Can you work these out from the model? Positions are in its coordinate system, mm. A direction names the side the tool comes from. Give positions to 0.01 mm unless a question says otherwise; leave off trailing zeros. Loops run counter-clockwise (first coordinate to the right, second up) from the corner with the lowest first, then second, coordinate; pieces in that order, holes last. Notation, with made-up numbers: M 17.25,-22 L 43.25,-22 A29 cw 43.25,-1 Z; hole C 48,69 d11. An arc over 180 degrees is marked long. One line per item, written item: value. Start each with the question number.
from build123d import *

# Parameters (mm, degrees)
F1_DEPTH    = 40.894
F2_R        = 5.08
F3_T1_DEPTH = 52.2452971888
F3_S5_W     = 5.08
F3_S5_H     = 5.08
F3_T6_DEPTH = 5.08
F4_W        = 7.728997618
F4_H        = 30.734
F4_W_2      = 7.9892426729
F5_DEPTH    = 5.08
F6_W        = 4.2550079525
F6_H        = 3.1596273184
F6_W_2      = 3.8497596979
F6_H_2      = 2.54
F7_DEPTH    = 39.37


# Not quite as in the source:
# - a fillet or chamfer that OpenCascade refuses, or shapes differently, is made with other operations: its cross-section is extruded or revolved along the edge and cut away or added
# - a feature of the source that left no trace in its solid (it failed there, or was rolled back) is left out


with BuildPart() as f1:
    # F0 (on Front) → F1 (new body)
    with BuildSketch(Plane.XZ):
        Polygon((45.526817441, 12.0578445494), (-38.0892679095, 12.0578445494), (-38.0892679095, -11.1563242972), (-38.0892679095, -32.5674526393), (-5.6345071644, -32.5674526393), (-5.6345071644, -24.228380993), (-31.1024785042, -24.228380993), (-31.1024785042, -11.1563242972), (45.526817441, -11.1563242972), align=None)
    extrude(amount=F1_DEPTH)

    # F2
    f2_edges = [f1.edges().sort_by_distance(p)[0] for p in [
        (45.526817, 0, 0.45076),
        (45.526817, -40.894, 0.45076),
        (-38.089268, 0, -10.254804),
        (3.718775, 0, 12.057845),
        (3.718775, -40.894, 12.057845),
        (45.526817, -20.447, 12.057845),
        (-38.089268, -20.447, 12.057845),
    ]]
    fillet(f2_edges, radius=F2_R)

    # F3: fillet of radius 5.08 on 1 edges, made by hand

    # F3_s2 → F3_t1 (cut)
    with BuildSketch(Plane.XY.offset(-45.2674526393)):
        with BuildLine():
            ThreePointArc((-38.0892679095, -35.814), (-36.601370358, -39.4061024484), (-33.0092679095, -40.894))
            Line((-33.0092679095, -40.894), (-38.0892679095, -40.894))
            Line((-38.0892679095, -40.894), (-38.0892679095, -35.814))
        make_face()
    extrude(amount=F3_T1_DEPTH, mode=Mode.SUBTRACT)


with BuildPart() as f3_tool4:
    # F3_s5 → F3_t6 (new body)
    with BuildSketch(Plane.YZ.offset(-33.0092679095)):
        with Locations((-38.354, 9.5178445494)):
            Rectangle(F3_S5_W, F3_S5_H)
    extrude(amount=-F3_T6_DEPTH)

    # F3_s7 → F3_t8 (revolve, cut)
    with BuildSketch(Plane(origin=(-33.0092679095, -35.814, 6.9778445494), x_dir=(0, 0.7071067812, -0.7071067812), z_dir=(0, 0.7071067812, 0.7071067812))):
        with BuildLine():
            ThreePointArc((0, -5.08), (5.08, 0), (0, 5.08))
            Line((0, 5.08), (0, -5.08))
        make_face()
    revolve(axis=Axis((-33.0092679095, -35.814, 6.9778445494), (-1, 0, 0)), mode=Mode.SUBTRACT)


with BuildPart() as f1_1:
    add(f1.part)

    # F3_t3: cut F3_tool4
    add(f3_tool4.part, mode=Mode.SUBTRACT)

    # F4 (on face) → F5 (join)
    with BuildSketch(Plane.XY.offset(12.0578445494)):
        with Locations((-22.0848601311, -20.447)):
            Rectangle(F4_W, F4_H)
        with Locations((19.4605253637, -20.447)):
            Rectangle(F4_W_2, F4_H)
    extrude(amount=F5_DEPTH)

    # F6 (on face) → F7 (cut)
    with BuildSketch(Plane.XZ.offset(35.814)):
        with Locations((-22.2941972315, 13.6376582086)):
            Rectangle(F6_W, F6_H)
        with Locations((19.4453038275, 13.3278445494)):
            Rectangle(F6_W_2, F6_H_2)
    extrude(amount=-F7_DEPTH, mode=Mode.SUBTRACT)


solid = f1_1.part
Q1. If we section it at D-D, the plane x = 4: Write out the boundary of the cut face in (y, z).
Q2. If we mould it in two halves opening along X, with no side actions, what happens to faces 4 (the face through (-20.167, -21, 14)), 5 (the face through (45.527, -20, -2)), 6 (the face through (-22, -5.08, 16))? For each: released by +X, released by -X, zero draft, split by the parting line, or undercut.
Q3. If we section it at C-C, the plane z = 11: Write out the boundary of the cut face in (x, y).
Q4. Which directions (+Z, -Z, +X, -X, +Y, -Y) give clear straight access to the entire face, cutting with the end or side of a thin tool? Please do faces 1 (the face through (-22, -21, 15.217)), 2 (the face through (-5.635, -20, -28)), 3 (the face through (19, -35.814, 15)).
Q5. If we section it at A-A, the plane y = -15.5: Write out the boundary of the cut face in (x, z), plus the area to 3 significant figures.
Q6. For P1, Ø12, axis at x = 9.5, y = -34.5, coming from the +Z side; P2, Ø1.5, axis at y = -27.5, z = 15.5, coming from the +X side; P3, Ø1.5, axis at y = -4, z = 11.5, coming from the -X side; P4, Ø4, axis at y = -17.5, z = 13.5, coming from the -X side, each with a flat end and sliding along its axis, tell me the tip position at first contact or that it passes through.
Q7. If we section it at B-B, the plane x = 22.5: Write out the boundary of the cut face in (y, z), plus the area to 3 significant figures.
Q8. I need wall thicknesses on line 1 along Z through (x, y) = (-21.5, -21); line 2 along X through (y, z) = (-16, 12.5); line 3 along Z through (x, y) = (-19, -19). Which ranges of each line are inside material? Lowest first, please.
Response:
1. outline: M -40.89,-11.16 L 0,-11.16 L 0,6.98 A5.08 ccw -5.08,12.06 L -35.81,12.06 A5.08 ccw -40.89,6.98 Z
2. face 4: undercut
2. face 5: released by +X
2. face 6: zero draft
3. outline: M -36.11,-35.81 A3.1 ccw -33.01,-38.92 L 40.45,-38.92 A3.1 ccw 43.55,-35.81 L 43.55,-5.08 A3.1 ccw 40.45,-1.98 L -33.01,-1.98 A3.1 ccw -36.11,-5.08 Z
4. face 1: +Y, -Y
4. face 2: -Z, +X, +Y, -Y
4. face 3: +Z, +X, -X, -Y
5. outline: M -38.09,-32.57 L -5.63,-32.57 L -5.63,-24.23 L -31.1,-24.23 L -31.1,-11.16 L 45.53,-11.16 L 45.53,6.98 A5.08 ccw 40.45,12.06 L 23.46,12.06 L 23.46,17.14 L 15.47,17.14 L 15.47,12.06 L -18.22,12.06 L -18.22,17.14 L -25.95,17.14 L -25.95,12.06 L -33.01,12.06 A5.08 ccw -38.09,6.98 Z; hole M -24.42,12.06 L -20.17,12.06 L -20.17,15.22 L -24.42,15.22 Z; hole M 17.52,12.06 L 21.37,12.06 L 21.37,14.6 L 17.52,14.6 Z
5. area: 2,350 mm^2
6. P1: z = 17.14
6. P2: x = 23.46
6. P3: x = -36.27
6. P4: x = -35.32
7. outline: M -40.89,-11.16 L 0,-11.16 L 0,6.98 A5.08 ccw -5.08,12.06 L -5.08,17.14 L -35.81,17.14 L -35.81,12.06 A5.08 ccw -40.89,6.98 Z
7. area: 1,090 mm^2
8. line 1: -32.57 to -24.23, -11.16 to 12.06, 15.22 to 17.14
8. line 2: -25.95 to -24.42, -20.17 to -18.22, 15.47 to 17.52, 21.37 to 23.46
8. line 3: -32.57 to -24.23, -11.16 to 17.14
